Read the model definition and answer for the solid it produces. Units are mm, in the model's axes. Face numbers are marked on the shaded views. A direction names the side the tool comes from. Coordinates: 2 decimals unless noted, no trailing zeros. Loops run counter-clockwise (first coordinate to the right, second up) from the corner with the lowest first, then second, coordinate; pieces in that order, holes last. Notation, with made-up numbers: M 29.25,61.25 L 61.25,61.25 A37 ccw 61.25,100.25 Z; hole C -31,32.5 d4. An arc over 180 degrees is marked long. One line per item, written item: value. Start each with the question number.
```python
from build123d import *

# Parameters (mm, degrees)
EXTRUDE2_DEPTH = 19.05


with BuildPart() as part:
    # Sketch2 → Extrude2 (new body)
    with BuildSketch(Plane(origin=(0, 0, 0), x_dir=(1, 0, 0), z_dir=(0, 1, 0))):
        with BuildLine():
            Line((0, 6.35), (0, 73.810967782))
            ThreePointArc((0, 73.810967782), (1.859871939, 78.301095843), (6.35, 80.160967782))
            Line((6.35, 80.160967782), (83.990365758, 80.160967782))
            ThreePointArc((83.990365758, 80.160967782), (88.480493819, 78.301095843), (90.340365758, 73.810967782))
            Line((90.340365758, 73.810967782), (90.340365758, 59.130483891))
            ThreePointArc((90.340365758, 59.130483891), (92.200237698, 54.640355831), (96.690365758, 52.780483891))
            Line((96.690365758, 52.780483891), (135.628548363, 52.780483891))
            ThreePointArc((135.628548363, 52.780483891), (140.118676423, 50.920611952), (141.978548363, 46.430483891))
            Line((141.978548363, 46.430483891), (141.978548363, 33.730483891))
            ThreePointArc((141.978548363, 33.730483891), (140.118676423, 29.240355831), (135.628548363, 27.380483891))
            Line((135.628548363, 27.380483891), (96.690365758, 27.380483891))
            ThreePointArc((96.690365758, 27.380483891), (92.200237698, 25.520611952), (90.340365758, 21.030483891))
            Line((90.340365758, 21.030483891), (90.340365758, 6.35))
            ThreePointArc((90.340365758, 6.35), (88.480493819, 1.859871939), (83.990365758, 0))
            Line((83.990365758, 0), (6.35, 0))
            ThreePointArc((6.35, 0), (1.859871939, 1.859871939), (0, 6.35))
        make_face()
    extrude(amount=-EXTRUDE2_DEPTH)


solid = part.part
```
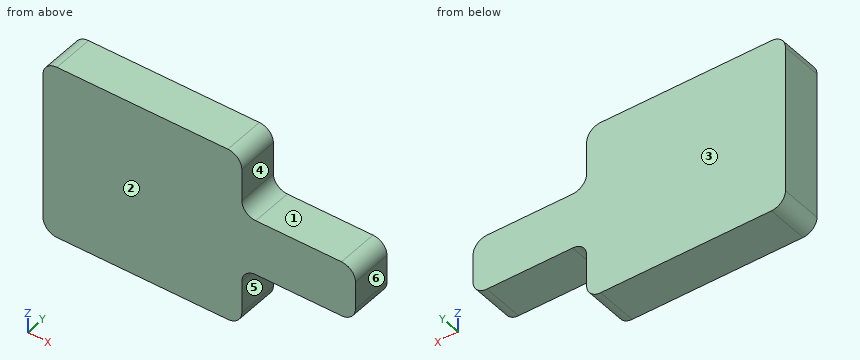
1) A tool of negligible diameter and unlimited length cuts with its end or side. For the marked faces 4, 5 and 6, from which of +Z, -Z, +X, -X, +Y, -Y can it reach the whole face along a straight path? Write none if from no direction.
2) Consider line 1 along Z through (x, y) = (120, -17); line 2 along X through (y, z) = (-2.5, -11); line 3 along X through (y, z) = (-4, -77). Determine where each line is inside the solid, lowest interval first.
3) Flat-ended cylindrical pins translate along their axes: pin 1 (5.5 mm diameter, centred on x = 119, y = -5.5, fed in from -Z); pin 2 (9.5 mm diameter, centred on x = 120.5, y = -8.5, fed in from +Z); pin 3 (6 mm diameter, centred on y = -9, z = -19.5, fed in from +X). Find the tip coordinate at first contact, or state that the pin passes through.
4) Section C-C (z = -11.5) is taken. Determine the outline of the cut face in (x, y).
5) For a pull along Y with two mould halves and no side action, classify the marked faces 1, 2 and 3 as released by +Y, released by -Y, zero draft, split by the parting line, or undercut.
6) Section B-B (x = 120) is taken. Determine the outline of the cut face in (y, z).
7) Section A-A (y = -17.25) is taken. Determine the outline of the cut face in (x, z), then the cut area to 3 significant figures.
Results found:
1. face 4: +Z, +X, +Y, -Y
1. face 5: -Z, +X, +Y, -Y
1. face 6: +Z, -Z, +X, +Y, -Y
2. line 1: z = -52.78 to -27.38
2. line 2: x = 0 to 90.34
2. line 3: x = 0.86 to 89.48
3. pin 1: stops at z = -52.78
3. pin 2: stops at z = -27.38
3. pin 3: stops at x = 90.51
4. outline: M 0,-19.05 L 90.34,-19.05 L 90.34,0 L 0,0 Z
5. face 1: zero draft
5. face 2: released by -Y
5. face 3: released by +Y
6. outline: M -19.05,-52.78 L 0,-52.78 L 0,-27.38 L -19.05,-27.38 Z
7. outline: M 0,-73.81 A6.35 ccw 6.35,-80.16 L 83.99,-80.16 A6.35 ccw 90.34,-73.81 L 90.34,-59.13 A6.35 cw 96.69,-52.78 L 135.63,-52.78 A6.35 ccw 141.98,-46.43 L 141.98,-33.73 A6.35 ccw 135.63,-27.38 L 96.69,-27.38 A6.35 cw 90.34,-21.03 L 90.34,-6.35 A6.35 ccw 83.99,0 L 6.35,0 A6.35 ccw 0,-6.35 Z
7. area: 8,520 mm²
